Answer from the drawing. Dimensions are ordinates in mm from the lowest x, y and z of the part. A direction names the side the tool comes from. Round coordinates to 2 decimals unless told otherwise and drop trailing zeros. Write each loop counter-clockwise with the first axis right and the second up, starting at its lowest first coordinate (ties: lowest second). Pieces come first, ordered by that corner, then holes. Notation, with made-up numbers: (-38, 3) - (6, 3) arc R19 cw to (6, 16) - close; hole circle Ø2 at (8.5, 30). An arc over 180 degrees is marked (long way). Answer as CSV lines item,"result". Start each with the question number.
1) Consider line 1 along X through (y, z) = (5, 8.5); line 2 along Y through (x, z) = (26.5, 1.4); line 3 along Z through (x, y) = (21, 23.25). Determine where each line is inside the solid, lowest interval first.
2) Find section C-C on x = 26.5. Determine the outline of the cut face in (y, z).
3) Find section D-D on y = 24. Determine the outline of the cut face in (x, z), then the cut area to 3 significant figures.
4) Find section B-B on y = 16.5. Determine the outline of the cut face in (x, z).
5) Each of these flat-tipped pins is pushed along its axis until it touches: pin 1 (1.2 mm diameter, centred on y = 24, z = 3.5, fed in from +X); pin 2 (2 mm diameter, centred on x = 26, z = 5, fed in from +Y); pin 3 (1.2 mm diameter, centred on y = 24, z = 3.5, fed in from -X). Where does it stop, or does it pass through?
6) Which of the six approach directions +Z, -Z, +X, -X, +Y, -Y give full straight-line access (tool end or side, diameter ignored) to the marked faces 4, 5, 6, 7 and 8?
7) For a pull along X with two mould halves and no side action, classify the marked faces 1, 2 and 3 as +X half, -X half, draft (parallel to the pull), parting line (faces both ways), or undercut.
8) Find section A-A on z = 6.5. Determine the outline of the cut face in (x, y), then the cut area to 3 significant figures.
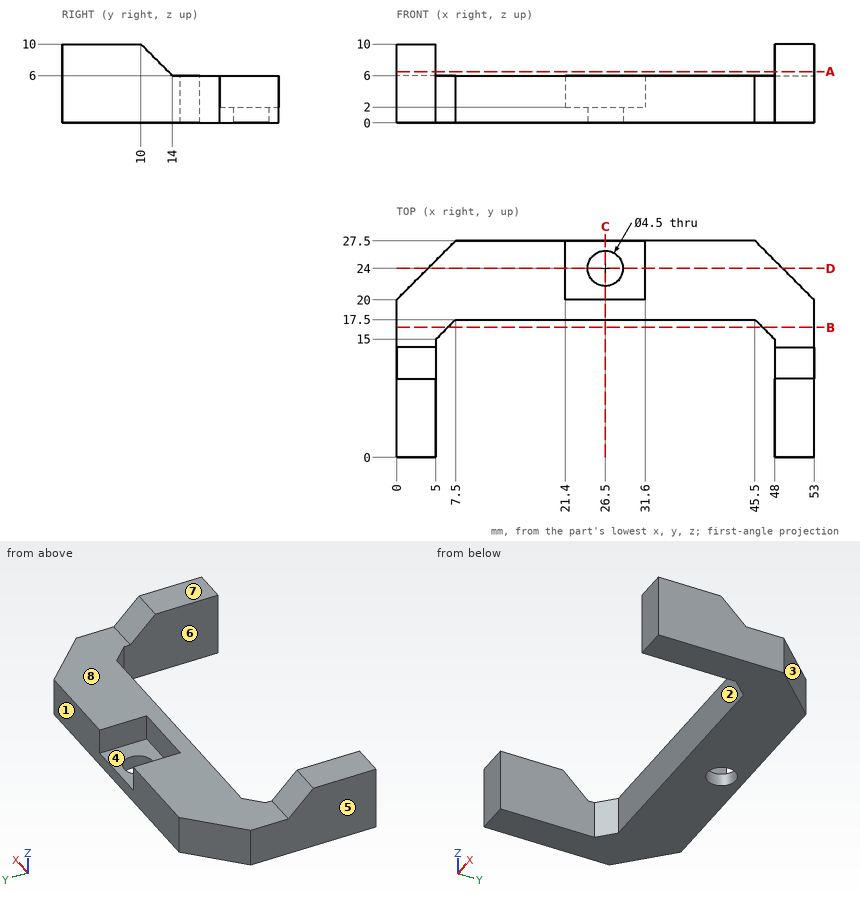
Check values:
1,line 1,"x = 0 to 5, 48 to 53"
1,line 2,"y = 17.5 to 21.75, 26.25 to 27.5"
1,line 3,"z = 0 to 6"
2,outline,"(17.5, 0) - (21.75, 0) - (21.75, 2) - (20, 2) - (20, 6) - (17.5, 6) - close; (26.25, 0) - (27.5, 0) - (27.5, 2) - (26.25, 2) - close"
3,outline,"(4, 0) - (24.25, 0) - (24.25, 2) - (21.4, 2) - (21.4, 6) - (4, 6) - close; (28.75, 0) - (49, 0) - (49, 6) - (31.6, 6) - (31.6, 2) - (28.75, 2) - close"
3,area,"220 mm^2"
4,outline,"(0, 0) - (6.5, 0) - (6.5, 6) - (0, 6) - close; (46.5, 0) - (53, 0) - (53, 6) - (46.5, 6) - close"
5,pin 1,"stops at x = 49.6"
5,pin 2,"stops at y = 20"
5,pin 3,"stops at x = 3.4"
6,face 4,"+Z, +Y"
6,face 5,"+Z, -Z, -X, +Y, -Y"
6,face 6,"+Z, -Z, -Y"
6,face 7,"+Z, +X, -X, +Y, -Y"
6,face 8,"+Z, +X, -X, +Y"
7,face 1,"draft"
7,face 2,"undercut"
7,face 3,"+X half"
8,outline,"(0, 0) - (5, 0) - (5, 13.5) - (0, 13.5) - close; (48, 0) - (53, 0) - (53, 13.5) - (48, 13.5) - close"
8,area,"135 mm^2"
